Read the model definition and answer for the solid it produces. Units are mm, in the model's axes. Coordinates: 2 decimals unless noted, no trailing zeros. One line per item, written item: value. Start each with the question number.
from build123d import *

# Parameters (mm, degrees)
SKETCH1_R                = 76.2
BOSS_EXTRUDE1_DEPTH      = 3.175
BOSS_EXTRUDE2_DEPTH      = 3.175
SKETCH3_R                = 4
BOSS_EXTRUDE3_DEPTH      = 0.0254
BOSS_EXTRUDE3_DEPTH_BACK = 6.35
CUT_EXTRUDE1_DEPTH       = 4.175
SKETCH6_W                = 72.50169985
SKETCH6_H                = 1.3335
CUT_EXTRUDE3_DEPTH       = 0.762
CIRPATTERN1_COUNT        = 4
SKETCH7_W                = 74.062567176
SKETCH7_H                = 1.3335
CUT_EXTRUDE4_DEPTH       = 0.762
CIRPATTERN2_COUNT        = 4
SKETCH8_R                = 1.905
CUT_EXTRUDE5_DEPTH       = 4.175


with BuildPart() as part:
    # Sketch1 → Boss-Extrude1 (new body)
    with BuildSketch(Plane(origin=(0, 0, 0), x_dir=(1, 0, 0), z_dir=(0, 1, 0))):
        Circle(SKETCH1_R)
    extrude(amount=BOSS_EXTRUDE1_DEPTH)

    # Sketch2 → Boss-Extrude2 (add)
    with BuildSketch(Plane(origin=(0, 3.175, 0), x_dir=(1, 0, 0), z_dir=(0, 1, 0))):
        with BuildLine():
            Line((-74.676, 1.524), (74.676, 1.524))
            ThreePointArc((74.676, 1.524), (76.2, 0), (74.676, -1.524))
            Line((74.676, -1.524), (-74.676, -1.524))
            ThreePointArc((-74.676, -1.524), (-76.2, 0), (-74.676, 1.524))
        make_face()
        with BuildLine():
            Line((1.4605, 74.7395), (1.4605, -74.7395))
            ThreePointArc((1.4605, -74.7395), (0, -76.2), (-1.4605, -74.7395))
            Line((-1.4605, -74.7395), (-1.4605, 74.7395))
            ThreePointArc((-1.4605, 74.7395), (0, 76.2), (1.4605, 74.7395))
        make_face()
    extrude(amount=BOSS_EXTRUDE2_DEPTH)

    # Sketch3 → Boss-Extrude3 (add, two sides)
    with BuildSketch(Plane(origin=(0, 6.35, 0), x_dir=(1, 0, 0), z_dir=(0, 1, 0))) as boss_extrude3_sk:
        Circle(SKETCH3_R)
    extrude(amount=BOSS_EXTRUDE3_DEPTH)
    extrude(boss_extrude3_sk.sketch, amount=-BOSS_EXTRUDE3_DEPTH_BACK)

    # Sketch4 → Cut-Extrude1 (cut, through all)
    with BuildSketch(Plane(origin=(0, 3.175, 0), x_dir=(1, 0, 0), z_dir=(0, 1, 0))):
        with BuildLine():
            Line((-7.8105, 7.874), (-39.5605, 7.874))
            Line((-39.5605, 7.874), (-63.009920838, 7.874))
            Line((-63.009920838, 7.874), (-66.208426571, 7.874))
            ThreePointArc((-66.208426571, 7.874), (-47.123731651, 47.168946779), (-7.8105, 66.215947586))
            Line((-7.8105, 66.215947586), (-7.8105, 63.017823588))
            Line((-7.8105, 63.017823588), (-7.8105, 7.874))
        make_face()
        with BuildLine():
            Line((7.874, 63.009920838), (7.874, 66.208426571))
            ThreePointArc((7.874, 66.208426571), (47.168946779, 47.123731651), (66.215947586, 7.8105))
            Line((66.215947586, 7.8105), (63.017823588, 7.8105))
            Line((63.017823588, 7.8105), (7.874, 7.8105))
            Line((7.874, 7.8105), (7.874, 39.5605))
            Line((7.874, 39.5605), (7.874, 63.009920838))
        make_face()
        with BuildLine():
            Line((63.009920838, -7.874), (66.208426571, -7.874))
            ThreePointArc((66.208426571, -7.874), (47.123731651, -47.168946779), (7.8105, -66.215947586))
            Line((7.8105, -66.215947586), (7.8105, -63.017823588))
            Line((7.8105, -63.017823588), (7.8105, -7.874))
            Line((7.8105, -7.874), (39.5605, -7.874))
            Line((39.5605, -7.874), (63.009920838, -7.874))
        make_face()
        with BuildLine():
            Line((-7.874, -63.009920838), (-7.874, -66.208426571))
            ThreePointArc((-7.874, -66.208426571), (-47.168946779, -47.123731651), (-66.215947586, -7.8105))
            Line((-66.215947586, -7.8105), (-63.017823588, -7.8105))
            Line((-63.017823588, -7.8105), (-7.874, -7.8105))
            Line((-7.874, -7.8105), (-7.874, -39.5605))
            Line((-7.874, -39.5605), (-7.874, -63.009920838))
        make_face()
    extrude(amount=-CUT_EXTRUDE1_DEPTH, mode=Mode.SUBTRACT)

    # Sketch6 → Cut-Extrude3 (cut)
    with BuildSketch(Plane.XY.offset(1.524)):
        with Locations((39.949150075, 3.84175)):
            Rectangle(SKETCH6_W, SKETCH6_H)
    cut_extrude3 = extrude(amount=-CUT_EXTRUDE3_DEPTH, mode=Mode.SUBTRACT)

    # CirPattern1: Cut-Extrude3 ×4 about axis
    cirpattern1_axis = Axis((0, 0, 0), (0, 1, 0))
    for i in range(1, CIRPATTERN1_COUNT):
        add(cut_extrude3.rotate(cirpattern1_axis, i * 360 / CIRPATTERN1_COUNT), mode=Mode.SUBTRACT)

    # Sketch7 → Cut-Extrude4 (cut)
    with BuildSketch(Plane(origin=(0, 0, -1.524), x_dir=(-1, 0, 0), z_dir=(0, 0, -1))):
        with Locations((-40.729583738, 3.84175)):
            Rectangle(SKETCH7_W, SKETCH7_H)
    cut_extrude4 = extrude(amount=-CUT_EXTRUDE4_DEPTH, mode=Mode.SUBTRACT)

    # CirPattern2: Cut-Extrude4 ×4 about axis
    cirpattern2_axis = Axis((0, 0, 0), (0, 1, 0))
    for i in range(1, CIRPATTERN2_COUNT):
        add(cut_extrude4.rotate(cirpattern2_axis, i * 360 / CIRPATTERN2_COUNT), mode=Mode.SUBTRACT)

    # Sketch8 → Cut-Extrude5 (cut, through all)
    with BuildSketch(Plane(origin=(0, 3.175, 0), x_dir=(1, 0, 0), z_dir=(0, 1, 0))):
        with Locations((-50.648644523, -50.648644523)):
            Circle(SKETCH8_R)
        with Locations((-50.648644523, 50.648644523)):
            Circle(SKETCH8_R)
        with Locations((50.648644523, 50.648644523)):
            Circle(SKETCH8_R)
        with Locations((50.648644523, -50.648644523)):
            Circle(SKETCH8_R)
    extrude(amount=-CUT_EXTRUDE5_DEPTH, mode=Mode.SUBTRACT)


solid = part.part
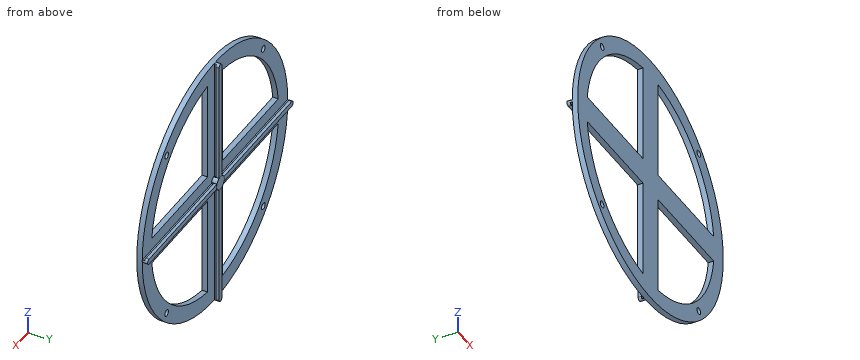
1) Flat-ended cylindrical pins translate along their axes: P1, Ø2, axis at y = 3.5, z = -28, coming from the -X side; P2, Ø0.7, axis at y = 4, z = -44.5, coming from the -X side; P3, Ø0.6, axis at x = -1.5, z = 43, coming from the -Y side; P4, Ø1, axis at x = 24.5, y = 1.5, coming from the -Z side. Find the tip coordinate at first contact, or state that the pin passes through.
2) Straight lines are drawn through the part: L1, parallel to Z at x = 15, y = 1.5; L2, parallel to Z at x = -14.5, y = 0.5; L3, parallel to X at y = 2, z = -8.5. For each, find the intervals that lie inside material, in ascending order.
3) Section A-A, the plane z = -36 is taken. State how many separate pieces and enclosed holes the cut face has, and give its area (3 significant figures).
Answer below:
1. P1: x = -71.24
1. P2: x = -0.76
1. P3: y = 0
1. P4: z = -72.32
2. L1: -74.71 to -64.97, -7.81 to 7.87, 64.97 to 74.71
2. L2: -74.81 to -65.08, -7.87 to 7.81, 65.08 to 74.81
2. L3: -75.72 to -66.13, -7.81 to 7.87, 66.13 to 75.72
3. separate pieces: 3
3. enclosed holes: 0
3. area: 127 mm2
